Source: CAD feature listing. Evaluate the final solid. Frame: model axes, mm. Face numbers are marked on the shaded views. Give positions to 0.01 mm unless a question says otherwise; leave off trailing zeros. Write each loop counter-clockwise with the first axis right and the second up, starting at its lowest first coordinate (ties: lowest second). Pieces come first, ordered by that corner, then holes. Notation, with made-up numbers: M 38.25,4.25 L 49.25,4.25 A20 cw 49.25,28.25 Z; hole C 0.25,78.5 d9. An arc over 180 degrees is marked long. Answer as a JSON object with one key per item and string values. Group by question number.
```python
from build123d import *

# Parameters (mm, degrees)
SKETCH619_W             = 480
SKETCH619_H             = 500
PAD295_DEPTH            = 70
SKETCH623_W             = 480
SKETCH623_H             = 70
PAD298_DEPTH            = 500
SKETCH620_W             = 50
SKETCH620_H             = 50
PAD294_DEPTH            = 490
SKETCH622_W             = 50
SKETCH622_H             = 50
PAD293_DEPTH            = 490
SKETCH621_W             = 50
SKETCH621_H             = 50
PAD296_DEPTH            = 490
SKETCH624_W             = 50
SKETCH624_H             = 50
PAD297_DEPTH            = 490
FILLET207_R             = 50
FILLET208_R             = 30
FILLET209_R             = 30
BODY125_PLACEMENT_ANGLE = 90


with BuildPart() as part:
    # Sketch619 → Pad295 (new body)
    with BuildSketch(Plane.XY):
        with Locations((240, 250)):
            Rectangle(SKETCH619_W, SKETCH619_H)
    extrude(amount=PAD295_DEPTH)

    # Sketch623 (on Face6 of Pad295) → Pad298 (join)
    with BuildSketch(Plane.XY.offset(70)):
        with Locations((240, 465)):
            Rectangle(SKETCH623_W, SKETCH623_H)
    extrude(amount=PAD298_DEPTH)

    # Sketch620 (on Face4 of Pad298) → Pad294 (join)
    with BuildSketch(Plane(origin=(0, 0, 0), x_dir=(1, 0, 0), z_dir=(0, 0, -1))):
        with Locations((75, -75)):
            Rectangle(SKETCH620_W, SKETCH620_H)
    extrude(amount=PAD294_DEPTH)

    # Sketch622 (on Face4 of Pad294) → Pad293 (join)
    with BuildSketch(Plane(origin=(0, 0, 0), x_dir=(1, 0, 0), z_dir=(0, 0, -1))):
        with Locations((405, -75)):
            Rectangle(SKETCH622_W, SKETCH622_H)
    extrude(amount=PAD293_DEPTH)

    # Sketch621 (on Face4 of Pad293) → Pad296 (join)
    with BuildSketch(Plane(origin=(0, 0, 0), x_dir=(1, 0, 0), z_dir=(0, 0, -1))):
        with Locations((75, -425)):
            Rectangle(SKETCH621_W, SKETCH621_H)
    extrude(amount=PAD296_DEPTH)

    # Sketch624 (on Face4 of Pad296) → Pad297 (join)
    with BuildSketch(Plane(origin=(0, 0, 0), x_dir=(1, 0, 0), z_dir=(0, 0, -1))):
        with Locations((405, -425)):
            Rectangle(SKETCH624_W, SKETCH624_H)
    extrude(amount=PAD297_DEPTH)

    # Fillet207
    fillet207_edges = [part.edges().sort_by_distance(p)[0] for p in [
        (240, 430, 570),
    ]]
    fillet(fillet207_edges, radius=FILLET207_R)

    # Fillet208
    fillet208_edges = [part.edges().sort_by_distance(p)[0] for p in [
        (240, 0, 70),
        (480, 215, 70),
        (0, 215, 70),
    ]]
    fillet(fillet208_edges, radius=FILLET208_R)

    # Fillet209
    fillet209_edges = [part.edges().sort_by_distance(p)[0] for p in [
        (480, 430, 295),
        (480, 444.644661, 555.355339),
        (0, 430, 295),
        (0, 444.644661, 555.355339),
    ]]
    fillet(fillet209_edges, radius=FILLET209_R)


with BuildPart() as part_1:
    # Body125 placement: moved
    add(part.part.moved(Location((3270, 2526, 462))).rotate(Axis((3270, 2526, 462), (0, 0, -1)), BODY125_PLACEMENT_ANGLE))


solid = part_1.part
```
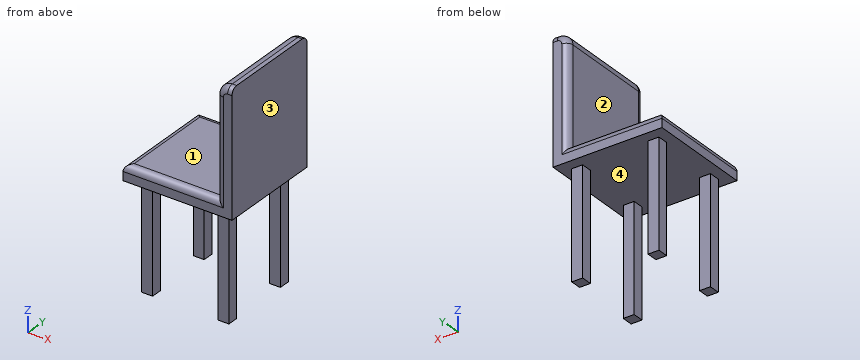
(1) Section A-A, the plane z = 96. Return loops of the section in (x, y).
(2) Section B-B, the plane x = 3330.5. Return loops of the section in (y, z).
(3) Ray query, L1, parallel to Y at x = 3363.5, z = 103; L2, parallel to X at y = 2124, z = 454; L3, parallel to Z at x = 3378, y = 2464. Return the intervals inside material, ascending. Write a range as [from, to].
(4) Pull-direction query (X, two-part tool) for the marked faces 1, 2, 3 and 4; classes: pulls with the +X half, pulls with the -X half, needs draft (parallel to the pull), parting line crosses it, or undercut.
(5) Contact query for flat-ended pins moving along their axis: pin 1 Ø25 at (x, z) = (3683, 271) entering from +Y; pin 2 Ø25 at (y, z) = (2454, 119.5) entering from -X; pin 3 Ø12 at (x, y) = (3517.5, 2412.5) entering from +Z. Output: stop coordinate, or through.
(6) Section D-D, the plane z = 629.5. Return loops of the section in (x, y).
(7) Section C-C, the plane y = 2412.5. Return loops of the section in (x, z), plus the area to 3 significant figures.
Reported:
{
 "1": {"outline": "M 3320,2096 L 3370,2096 L 3370,2146 L 3320,2146 Z; M 3320,2426 L 3370,2426 L 3370,2476 L 3320,2476 Z; M 3670,2096 L 3720,2096 L 3720,2146 L 3670,2146 Z; M 3670,2426 L 3720,2426 L 3720,2476 L 3670,2476 Z"},
 "2": {"outline": "M 2046,462 L 2096,462 L 2096,-28 L 2146,-28 L 2146,462 L 2426,462 L 2426,-28 L 2476,-28 L 2476,462 L 2526,462 L 2526,502 A30 ccw 2496,532 L 2076,532 A30 ccw 2046,502 Z"},
 "3": {"L1": "y = [2096, 2146], [2426, 2476]", "L2": "x = [3320, 3370], [3670, 3720]", "L3": "z = [462, 532]"},
 "4": {"face 1": "needs draft", "face 2": "pulls with the -X half", "face 3": "pulls with the +X half", "face 4": "undercut"},
 "5": {"pin 1": "stops at y = 2476", "pin 2": "stops at x = 3320", "pin 3": "stops at z = 532"},
 "6": {"outline": "M 3700,2076 A30 ccw 3730,2046 L 3770,2046 L 3770,2526 L 3730,2526 A30 ccw 3700,2496 Z"},
 "7": {"outline": "M 3270,462 L 3770,462 L 3770,1032 L 3750,1032 A50 ccw 3700,982 L 3700,532 L 3300,532 A30 ccw 3270,502 Z", "area": "69,300 mm2"}
}
